```python
from build123d import *

# Parameters (mm, degrees)
SKETCH_1_W                     = 80
SKETCH_1_H                     = 60
EXTRUDE_1_DEPTH                = 2
SKETCH_2_W                     = 74
SKETCH_2_H                     = 54
EXTRUDE_2_DEPTH                = 1
HOLE_WIZARD_M3_5_1_D           = 2.9
HOLE_WIZARD_M3_5_1_DEPTH       = 8.8
HOLE_WIZARD_M3_5_1_CSINK_D     = 3.55
HOLE_WIZARD_M3_5_1_CSINK_ANGLE = 90
HOLE_WIZARD_M3_5_1_TIP         = 0.871247898


with BuildPart() as part:
    # 草图1 → 凸台-拉伸1 (new body)
    with BuildSketch(Plane(origin=(0, 0, 0), x_dir=(1, 0, 0), z_dir=(0, 1, 0))):
        with Locations((40, 30)):
            Rectangle(SKETCH_1_W, SKETCH_1_H)
    extrude(amount=EXTRUDE_1_DEPTH)

    # 草图2 → 凸台-拉伸2 (add)
    with BuildSketch(Plane(origin=(0, 2, 0), x_dir=(1, 0, 0), z_dir=(0, 1, 0))):
        Polygon((80, 60), (0, 60), (0, 57), (0, 0), (80, 0), align=None)
        with Locations((40, 30)):
            Rectangle(SKETCH_2_W, SKETCH_2_H, mode=Mode.SUBTRACT)
    extrude(amount=EXTRUDE_2_DEPTH)

    # M3.5 螺纹孔1
    with Locations(Plane.XZ):
        with Locations((5.5, -3), (74.5, -3), (12.5, -52), (67.5, -52)):
            CounterSinkHole(HOLE_WIZARD_M3_5_1_D / 2, HOLE_WIZARD_M3_5_1_CSINK_D / 2, depth=HOLE_WIZARD_M3_5_1_DEPTH, counter_sink_angle=HOLE_WIZARD_M3_5_1_CSINK_ANGLE)
            with Locations((0, 0, -(HOLE_WIZARD_M3_5_1_DEPTH + HOLE_WIZARD_M3_5_1_TIP / 2))):  # 118° drill point
                Cone(0, HOLE_WIZARD_M3_5_1_D / 2, HOLE_WIZARD_M3_5_1_TIP, mode=Mode.SUBTRACT)


solid = part.part
```
Source: CAD feature listing. Evaluate the final solid. Frame: model axes, mm. A direction names the side the tool comes from. Give positions to 0.01 mm unless a question says otherwise; leave off trailing zeros. Loops run counter-clockwise (first coordinate to the right, second up) from the corner with the lowest first, then second, coordinate; pieces in that order, holes last. Notation, with made-up numbers: (32, 45.5) - (68, 45.5) arc R20 cw to (68, 63.5) - close; hole circle Ø11 at (-26.75, 76.25). An arc over 180 degrees is marked (long way). Use CSV: the item, a comma, the result in double quotes.
1) Set-up query: faces 1 (the cylindrical face through (12.814, 1.174, -53.416)), 2 (the flat face through (39, 2, -30)). Return all of +Z, -Z, +X, -X, +Y, -Y with unobstructed straight access to the full face (end or side cutting, diameter ignored); none if empty.
Worked out:
face 1,"+Y, -Y"
face 2,"+Y"
2) Line query: line 1 (X direction, y = 0.9, z = -52); line 2 (X direction, y = 1.5, z = -3); line 3 (X direction, y = 2.85, z = -11). Output: solid intervals per line, ascending.
Worked out:
line 1,"x = 0 to 11.05, 13.95 to 66.05, 68.95 to 80"
line 2,"x = 0 to 4.05, 6.95 to 73.05, 75.95 to 80"
line 3,"x = 0 to 3, 77 to 80"
3) Cut plane C-C (y = 2.5). Output: boundary loops of the cut face in (x, z), and give its area (3 significant figures).
Worked out:
outline,"(0, -60) - (80, -60) - (80, 0) - (0, 0) - close; hole (3, -57) - (77, -57) - (77, -3) - (75.95, -3) arc R1.45 ccw to (73.05, -3) - (6.95, -3) arc R1.45 ccw to (4.05, -3) - (3, -3) - close"
area,"797 mm^2"
4) Cut plane A-A (x = 67.5). Output: boundary loops of the cut face in (y, z) (3 decimals), and give its area (3 significant figures).
Worked out:
outline,"(0, -60) - (3, -60) - (3, -57) - (2, -57) - (2, -53.45) - (0.325, -53.45) - (0, -53.775) - close; (0, -50.225) - (0.325, -50.55) - (2, -50.55) - (2, -3) - (3, -3) - (3, 0) - (0, 0) - close"
area,"120 mm^2"
5) Pin query (flat end, axial travel): P1, Ø4.5, axis at x = 67.5, z = -52, coming from the +Y side; P2, Ø2.5, axis at x = 12.5, z = -52, coming from the +Y side; P3, Ø1.5, axis at x = 26, y = 2, coming from the +Z side. Return the tip coordinate at first contact, or that it passes through.
Worked out:
P1,"stops at y = 2"
P2,"passes through"
P3,"stops at z = 0"
6) Cut plane B-B (z = -52). Output: boundary loops of the cut face in (x, y) (3 decimals).
Worked out:
outline,"(0, 0) - (10.725, 0) - (11.05, 0.325) - (11.05, 2) - (3, 2) - (3, 3) - (0, 3) - close; (13.95, 0.325) - (14.275, 0) - (65.725, 0) - (66.05, 0.325) - (66.05, 2) - (13.95, 2) - close; (68.95, 0.325) - (69.275, 0) - (80, 0) - (80, 3) - (77, 3) - (77, 2) - (68.95, 2) - close"
7) Mould query, pull axis Z, two halves, no side actions, for faces 3 (the flat face through (80, 1, -30)), 4 (the flat face through (41, 1, -60)), 5 (the cylindrical face through (68.65, 1.17, -52.88)). Classes: +Z half, -Z half, draft (parallel to the pull), parting line (faces both ways), or undercut.
Worked out:
face 3,"draft"
face 4,"-Z half"
face 5,"undercut"
8) Cut plane D-D (z = -39). Output: boundary loops of the cut face in (x, y), and give its area (3 significant figures).
Worked out:
outline,"(0, 0) - (80, 0) - (80, 3) - (77, 3) - (77, 2) - (3, 2) - (3, 3) - (0, 3) - close"
area,"166 mm^2"
